Input: part model. Units: mm. Frame: model coordinates. Face numbers are marked on the shaded views. A direction names the side the tool comes from. Coordinates: 2 decimals unless noted, no trailing zeros. Write each loop counter-clockwise with the first axis right and the second up, starting at its lowest first coordinate (ties: lowest second). Pieces come first, ordered by that corner, then holes. Notation, with made-up numbers: M 56,-16.5 L 71,-16.5 A14 ccw 71,-12.5 Z; hole C -32.5,-14.75 d8. An arc over 180 degrees is marked long. Write each question's results on one line, items separated by ' | '. Start each with the question number.
1. Pull-direction query (Y, two-part tool) for the marked faces 6, 7 and 8; classes: +Y half, -Y half, draft (parallel to the pull), parting line (faces both ways), or undercut.
2. Section query D-D, the plane x = 21.75. Output: boundary loops of the cut face in (y, z).
3. Section query A-A, the plane z = 1.5. Count the separate pieces of the cut face and the enclosed holes in it, and give its area (3 significant figures).
4. Section query C-C, the plane z = 5.75. Output: boundary loops of the cut face in (x, y).
5. Section query B-B, the plane y = 12.5. Output: boundary loops of the cut face in (x, z), and give its area (3 significant figures).
6. Set-up query: the marked faces 1, 2, 3, 4 and 5. Return all of +Z, -Z, +X, -X, +Y, -Y with unobstructed straight access to the full face (end or side cutting, diameter ignored); none if empty.
7. Ray query, probe 1 along Y at (x, z) = (37.7, 0.45); probe 2 along Z at (x, y) = (14, 27); probe 3 along X at (y, z) = (38, 3). Return the intervals inside material, ascending.
8. First-contact query: pin 1 (1.2 mm diameter, centred on x = 37.7, y = 37.7, fed in from -Z); pin 2 (1.2 mm diameter, centred on x = 22.5, z = 3, fed in from -Y); pin 3 (0.9 mm diameter, centred on x = 33.5, y = 11.5, fed in from +Z); pin 4 (1.5 mm diameter, centred on y = 2, z = 3, fed in from +X). Flat tips, straight axial feed; report the tip coordinate or a pass-through.
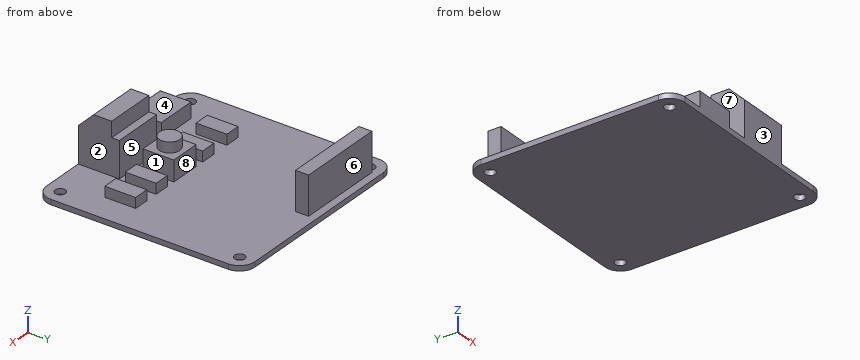
```python
from build123d import *

# Parameters (mm, degrees)
ESQUISSE1_W             = 40.5
ESQUISSE1_H             = 40.5
ESQUISSE1_R             = 1
BOSS_EXTRU_1_DEPTH      = 1
CONG_1_R                = 3
ESQUISSE2_W             = 10
ESQUISSE2_H             = 8
BOSS_EXTRU_2_DEPTH      = 10
ESQUISSE3_W             = 3
ESQUISSE3_H             = 1.5
ENL_V_MAT_EXTRU_1_DEPTH = 10
ESQUISSE4_W             = 8
ESQUISSE4_H             = 6
BOSS_EXTRU_3_DEPTH      = 3
ESQUISSE5_W             = 3
ESQUISSE5_H             = 6
BOSS_EXTRU_4_DEPTH      = 2
ESQUISSE6_W             = 6
ESQUISSE6_H             = 6
BOSS_EXTRU_5_DEPTH      = 4
ESQUISSE7_R             = 2
BOSS_EXTRU_6_DEPTH      = 2
ESQUISSE8_W             = 17
ESQUISSE8_H             = 2.54
BOSS_EXTRU_7_DEPTH      = 7.5


with BuildPart() as part:
    # Esquisse1 → Boss.-Extru.1 (new body)
    with BuildSketch(Plane.XY):
        with Locations((20.25, 20.25)):
            Rectangle(ESQUISSE1_W, ESQUISSE1_H)
        with Locations((37.7, 37.7)):
            Circle(ESQUISSE1_R, mode=Mode.SUBTRACT)
        with Locations((37.7, 2.8)):
            Circle(ESQUISSE1_R, mode=Mode.SUBTRACT)
        with Locations((2.8, 2.8)):
            Circle(ESQUISSE1_R, mode=Mode.SUBTRACT)
        with Locations((2.8, 37.7)):
            Circle(ESQUISSE1_R, mode=Mode.SUBTRACT)
    extrude(amount=BOSS_EXTRU_1_DEPTH)

    # Congé1
    cong_1_edges = [part.edges().sort_by_distance(p)[0] for p in [
        (0, 40.5, 0.5),
        (40.5, 40.5, 0.5),
        (40.5, 0, 0.5),
        (0, 0, 0.5),
    ]]
    fillet(cong_1_edges, radius=CONG_1_R)

    # Esquisse2 → Boss.-Extru.2 (add)
    with BuildSketch(Plane.XY.offset(1)):
        with Locations((24, 4)):
            Rectangle(ESQUISSE2_W, ESQUISSE2_H)
    extrude(amount=BOSS_EXTRU_2_DEPTH)

    # Esquisse3 → Enlèv. mat.-Extru.1 (cut)
    with BuildSketch(Plane(origin=(29, 0, 0), x_dir=(0, 0, -1), z_dir=(1, 0, 0))):
        Polygon((-8, 0), (-11, 3), (-11, 0), align=None)
        with Locations((-9.5, 7.25)):
            Rectangle(ESQUISSE3_W, ESQUISSE3_H)
    extrude(amount=-ENL_V_MAT_EXTRU_1_DEPTH, mode=Mode.SUBTRACT)

    # Esquisse4 → Boss.-Extru.3 (add)
    with BuildSketch(Plane.XY.offset(1)):
        with Locations((11, 3)):
            Rectangle(ESQUISSE4_W, ESQUISSE4_H)
    extrude(amount=BOSS_EXTRU_3_DEPTH)

    # Esquisse5 → Boss.-Extru.4 (add)
    with BuildSketch(Plane.XY.offset(1)):
        with Locations((9, 12.5)):
            Rectangle(ESQUISSE5_W, ESQUISSE5_H)
        with Locations((15.5, 12.5)):
            Rectangle(ESQUISSE5_W, ESQUISSE5_H)
        with Locations((28, 12.5)):
            Rectangle(ESQUISSE5_W, ESQUISSE5_H)
        with Locations((33.5, 12.5)):
            Rectangle(ESQUISSE5_W, ESQUISSE5_H)
    extrude(amount=BOSS_EXTRU_4_DEPTH)

    # Esquisse6 → Boss.-Extru.5 (add)
    with BuildSketch(Plane.XY.offset(1)):
        with Locations((21.75, 12.5)):
            Rectangle(ESQUISSE6_W, ESQUISSE6_H)
    extrude(amount=BOSS_EXTRU_5_DEPTH)

    # Esquisse7 → Boss.-Extru.6 (add)
    with BuildSketch(Plane.XY.offset(5)):
        with Locations((21.75, 12.5)):
            Circle(ESQUISSE7_R)
    extrude(amount=BOSS_EXTRU_6_DEPTH)

    # Esquisse8 → Boss.-Extru.7 (add)
    with BuildSketch(Plane.XY.offset(1)):
        with Locations((12.5, 37.73)):
            Rectangle(ESQUISSE8_W, ESQUISSE8_H)
    extrude(amount=BOSS_EXTRU_7_DEPTH)


solid = part.part
```
Answer:
1) face 6: +Y half | face 7: draft | face 8: undercut
2) outline: M 0,0 L 40.5,0 L 40.5,1 L 15.5,1 L 15.5,5 L 14.5,5 L 14.5,7 L 10.5,7 L 10.5,5 L 9.5,5 L 9.5,1 L 8,1 L 8,8 L 6.5,8 L 6.5,11 L 3,11 L 0,8 Z
3) separate pieces: 8 | enclosed holes: 0 | area: 279 mm^2
4) outline: M 4,36.46 L 21,36.46 L 21,39 L 4,39 Z; M 19,0 L 29,0 L 29,8 L 19,8 Z; C 21.75,12.5 d4
5) outline: M 0,0 L 40.5,0 L 40.5,1 L 35,1 L 35,3 L 32,3 L 32,1 L 29.5,1 L 29.5,3 L 26.5,3 L 26.5,1 L 24.75,1 L 24.75,5 L 23.75,5 L 23.75,7 L 19.75,7 L 19.75,5 L 18.75,5 L 18.75,1 L 17,1 L 17,3 L 14,3 L 14,1 L 10.5,1 L 10.5,3 L 7.5,3 L 7.5,1 L 0,1 Z | area: 96.5 mm^2
6) face 1: +Z, +Y | face 2: +Z, +X, -Y | face 3: +Z, -Z, +X, -X, -Y | face 4: +Z, -X, -Y | face 5: +Z, +X, -X
7) probe 1: 0.01 to 1.8, 3.8 to 36.7, 38.7 to 40.49 | probe 2: 0 to 1 | probe 3: 4 to 21
8) pin 1: through | pin 2: y = 0 | pin 3: z = 3 | pin 4: x = 29
